The figure shows three views and two pictorial views of one solid part (mm, origin at its lowest corner). Answer the questions. Round coordinates to 2 decimals unless told otherwise and drop trailing zeros. Order: outer loops, then holes, each group sorted by start corner. A loop starts at its lowest first (then second) coordinate and runs counter-clockwise, first axis right, second up. Notation, with made-up numbers: (42.25, 20.25) - (99.25, 20.25) arc R12 cw to (99.25, 40.25) - close; hole circle Ø8 at (89, 11). An arc over 180 degrees is marked (long way). Answer in a Markdown table with one row per item.
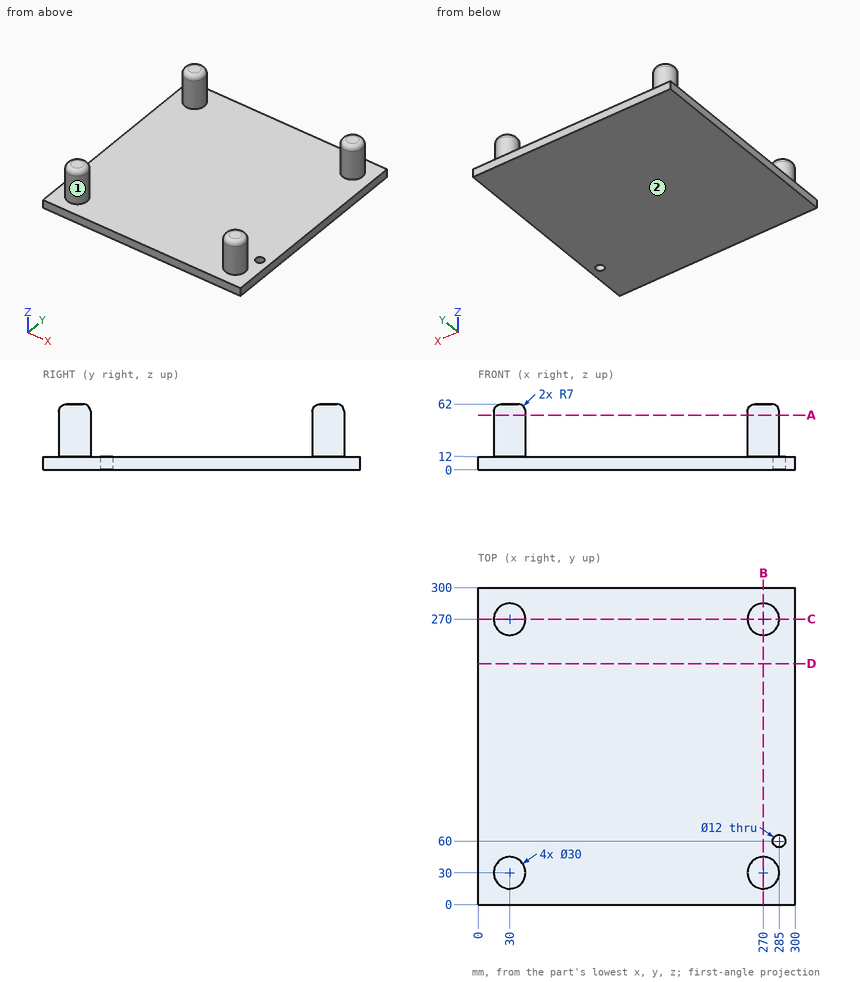
1) Find section B-B, the plane x = 270. Give the vertices of the cut face in (y, z), then the cut area to 3 significant figures.
Filled in:
| item | result |
|---|---|
| outline | (0, 0) - (300, 0) - (300, 12) - (285, 12) - (285, 55) arc R7 ccw to (278, 62) - (262, 62) arc R7 ccw to (255, 55) - (255, 12) - (45, 12) - (45, 55) arc R7 ccw to (38, 62) - (22, 62) arc R7 ccw to (15, 55) - (15, 12) - (0, 12) - close |
| area | 6,560 mm^2 |
2) The mould has two halves that part along X. Classify the marked faces 1 and 2: released by +X, released by -X, zero draft, split by the parting line, or undercut.
Filled in:
| item | result |
|---|---|
| face 1 | undercut |
| face 2 | zero draft |
3) Each of these flat-tipped pins is pushed along its axis until it touches: pin 1 (5 mm diameter, centred on x = 93, y = 123.5, fed in from +Z); pin 2 (3 mm diameter, centred on y = 30, z = 41.5, fed in from +X). Where does it stop, or does it pass through?
Filled in:
| item | result |
|---|---|
| pin 1 | stops at z = 12 |
| pin 2 | stops at x = 285 |
4) Find section D-D, the plane y = 228. Give the vertices of the cut face in (x, z).
Filled in:
| item | result |
|---|---|
| outline | (0, 0) - (300, 0) - (300, 12) - (0, 12) - close |
5) Find section A-A, the plane z = 51.5. Give the vertices of the cut face in (x, y), then the cut area to 3 significant figures.
Filled in:
| item | result |
|---|---|
| outline | circle Ø30 at (30, 30); circle Ø30 at (30, 270); circle Ø30 at (270, 30); circle Ø30 at (270, 270) |
| area | 2,830 mm^2 |
6) Find the intervals of material crossed by probe 1 along Y at (x, z) = (285, 4); probe 2 along X at (y, z) = (30.5, 50); probe 3 along Z at (x, y) = (285.5, 166), in increasing order. Write a range as from..to.
Filled in:
| item | result |
|---|---|
| probe 1 | y = 0..54, 66..300 |
| probe 2 | x = 15.01..44.99, 255.01..284.99 |
| probe 3 | z = 0..12 |
